Source: CAD feature listing. Evaluate the final solid. Frame: model axes, mm. A direction names the side the tool comes from. Give positions to 0.01 mm unless a question says otherwise; leave off trailing zeros. Write each loop counter-clockwise with the first axis right and the second up, starting at its lowest first coordinate (ties: lowest second). Pieces come first, ordered by that corner, then holes.
```python
from build123d import *

# Parameters (mm, degrees)
RESSALTO_EXTRUS_O1_DEPTH             = 3
ESBO_O2_R                            = 4
CORTE_EXTRUS_O1_DEPTH                = 10
ESCAREADO_PARA_SFHCS_M31_AT_2_COUNT  = 2
ESCAREADO_PARA_SFHCS_M31_AT_2_PITCH  = 110.302460898
ESCAREADO_PARA_SFHCS_M31_AT_3_COUNT  = 2
ESCAREADO_PARA_SFHCS_M31_AT_3_PITCH  = 130.842986965
ESCAREADO_PARA_SFHCS_M31_AT_4_COUNT  = 2
ESCAREADO_PARA_SFHCS_M31_AT_4_PITCH  = 67
ESCAREADO_PARA_SFHCS_M31_AT_5_COUNT  = 2
ESCAREADO_PARA_SFHCS_M31_AT_5_PITCH  = 132.532334398
ESCAREADO_PARA_SFHCS_M31_AT_6_COUNT  = 2
ESCAREADO_PARA_SFHCS_M31_AT_6_PITCH  = 175.070818678
ESCAREADO_PARA_SFHCS_M31_AT_7_COUNT  = 2
ESCAREADO_PARA_SFHCS_M31_AT_7_PITCH  = 213.572320447
ESCAREADO_PARA_SFHCS_M31_AT_8_COUNT  = 2
ESCAREADO_PARA_SFHCS_M31_AT_8_PITCH  = 243.433045731
ESCAREADO_PARA_SFHCS_M31_AT_9_COUNT  = 2
ESCAREADO_PARA_SFHCS_M31_AT_9_PITCH  = 142.710342559
ESCAREADO_PARA_SFHCS_M41_AT_2_COUNT  = 2
ESCAREADO_PARA_SFHCS_M41_AT_2_PITCH  = 40
ESCAREADO_PARA_SFHCS_M41_AT_3_COUNT  = 2
ESCAREADO_PARA_SFHCS_M41_AT_3_PITCH  = 46.75082887
ESCAREADO_PARA_SFHCS_M41_AT_4_COUNT  = 2
ESCAREADO_PARA_SFHCS_M41_AT_4_PITCH  = 24.2
ESCAREADO_PARA_SFHCS_M41_AT_5_COUNT  = 2
ESCAREADO_PARA_SFHCS_M41_AT_5_PITCH  = 58.077850276
ESCAREADO_PARA_SFHCS_M41_AT_6_COUNT  = 2
ESCAREADO_PARA_SFHCS_M41_AT_6_PITCH  = 43.020334562
ESCAREADO_PARA_SFHCS_M41_AT_7_COUNT  = 2
ESCAREADO_PARA_SFHCS_M41_AT_7_PITCH  = 136.807623633
ESCAREADO_PARA_SFHCS_M41_AT_8_COUNT  = 2
ESCAREADO_PARA_SFHCS_M41_AT_8_PITCH  = 139.831145131
ESCAREADO_PARA_SFHCS_M41_AT_9_COUNT  = 2
ESCAREADO_PARA_SFHCS_M41_AT_9_PITCH  = 173.161507104
ESCAREADO_PARA_SFHCS_M41_AT_10_COUNT = 2
ESCAREADO_PARA_SFHCS_M41_AT_10_PITCH = 170.775968029
ESCAREADO_PARA_SFHCS_M41_AT_11_COUNT = 2
ESCAREADO_PARA_SFHCS_M41_AT_11_PITCH = 332.816318971
ESCAREADO_PARA_SFHCS_M41_AT_12_COUNT = 2
ESCAREADO_PARA_SFHCS_M41_AT_12_PITCH = 333.669600313
ESCAREADO_PARA_SFHCS_M41_AT_13_COUNT = 2
ESCAREADO_PARA_SFHCS_M41_AT_13_PITCH = 373.827719057
ESCAREADO_PARA_SFHCS_M41_AT_14_COUNT = 2
ESCAREADO_PARA_SFHCS_M41_AT_14_PITCH = 373.066299115
ESBO_O9_W                            = 8
ESBO_O9_H                            = 4
CORTE_EXTRUS_O2_DEPTH                = 230.077241914


with BuildPart() as part:
    # Esboço1 → Ressalto-extrusão1 (new body)
    with BuildSketch(Plane(origin=(0, 0, 0), x_dir=(1, 0, 0), z_dir=(0, 1, 0))):
        with BuildLine():
            Line((-2.5, 209.375), (2.5, 209.375))
            ThreePointArc((2.5, 209.375), (3.560660172, 209.814339828), (4, 210.875))
            Line((4, 210.875), (4, 213.875))
            ThreePointArc((4, 213.875), (4.439339828, 214.935660172), (5.5, 215.375))
            Line((5.5, 215.375), (21, 215.375))
            ThreePointArc((21, 215.375), (23.121320344, 214.496320344), (24, 212.375))
            Line((24, 212.375), (24, 187.375))
            Line((24, 187.375), (35.808734273, 177.675))
            ThreePointArc((35.808734273, 177.675), (37.1583493, 172.791760303), (33.015886264, 169.875))
            Line((33.015886264, 169.875), (31, 169.875))
            ThreePointArc((31, 169.875), (28.878679656, 168.996320344), (28, 166.875))
            Line((28, 166.875), (28, 155.375))
            Line((28, 155.375), (66.5, 111.375))
            Line((66.5, 111.375), (59.5, -111.375))
            Line((59.5, -111.375), (48, -117.875))
            Line((48, -117.875), (29, -154.770121629))
            Line((29, -154.770121629), (29, -166.370121629))
            ThreePointArc((29, -166.370121629), (29.878679656, -168.491441972), (32, -169.370121629))
            Line((32, -169.370121629), (32.371701685, -169.370121629))
            ThreePointArc((32.371701685, -169.370121629), (36.448422746, -171.9647751), (35.823953384, -176.756634787))
            Line((35.823953384, -176.756634787), (22.5, -192.691999769))
            Line((22.5, -192.691999769), (22.5, -216.191999769))
            ThreePointArc((22.5, -216.191999769), (21.621320344, -218.313320113), (19.5, -219.191999769))
            Line((19.5, -219.191999769), (-19.5, -219.191999769))
            ThreePointArc((-19.5, -219.191999769), (-21.621320344, -218.313320113), (-22.5, -216.191999769))
            Line((-22.5, -216.191999769), (-22.5, -192.691999769))
            Line((-22.5, -192.691999769), (-35.823953384, -176.756634787))
            ThreePointArc((-35.823953384, -176.756634787), (-36.448422746, -171.9647751), (-32.371701685, -169.370121629))
            Line((-32.371701685, -169.370121629), (-32, -169.370121629))
            ThreePointArc((-32, -169.370121629), (-29.878679656, -168.491441972), (-29, -166.370121629))
            Line((-29, -166.370121629), (-29, -154.770121629))
            Line((-29, -154.770121629), (-48, -117.875))
            Line((-48, -117.875), (-59.5, -111.375))
            Line((-59.5, -111.375), (-66.5, 111.375))
            Line((-66.5, 111.375), (-28, 155.375))
            Line((-28, 155.375), (-28, 166.875))
            ThreePointArc((-28, 166.875), (-28.878679656, 168.996320344), (-31, 169.875))
            Line((-31, 169.875), (-33.015886264, 169.875))
            ThreePointArc((-33.015886264, 169.875), (-37.1583493, 172.791760303), (-35.808734273, 177.675))
            Line((-35.808734273, 177.675), (-24, 187.375))
            Line((-24, 187.375), (-24, 212.375))
            ThreePointArc((-24, 212.375), (-23.121320344, 214.496320344), (-21, 215.375))
            Line((-21, 215.375), (-5.5, 215.375))
            ThreePointArc((-5.5, 215.375), (-4.439339828, 214.935660172), (-4, 213.875))
            Line((-4, 213.875), (-4, 210.875))
            ThreePointArc((-4, 210.875), (-3.560660172, 209.814339828), (-2.5, 209.375))
        make_face()
    extrude(amount=RESSALTO_EXTRUS_O1_DEPTH)

    # Esboço2 → Corte-extrusão1 (cut)
    with BuildSketch(Plane(origin=(0, 3, 0), x_dir=(1, 0, 0), z_dir=(0, 1, 0))):
        with Locations(Location((-45, -79.191999769, 0), (0, 0, 270))):
            Circle(ESBO_O2_R)
        with Locations(Location((45, -79.191999769, 0), (0, 0, 270))):
            Circle(ESBO_O2_R)
        with Locations(Location((45, 110.808000231, 0), (0, 0, 270))):
            Circle(ESBO_O2_R)
        with Locations(Location((-45, 110.808000231, 0), (0, 0, 270))):
            Circle(ESBO_O2_R)
    extrude(amount=-CORTE_EXTRUS_O1_DEPTH, mode=Mode.SUBTRACT)

    # Esboço6 → Escareado para SFHCS M31 (revolve, cut)
    with BuildSketch(Plane(origin=(55.151230449, 0, 106.491941439), x_dir=(0, 0, -1), z_dir=(1, 0, 0))):
        Polygon((0, 0), (0, 3), (1.7, 3), (1.7, 1.66), (3.36, 0), align=None)
    escareado_para_sfhcs_m31 = revolve(axis=Axis((55.151230449, -6.35, 106.491941439), (0, 1, 0)), mode=Mode.SUBTRACT)

    # Escareado para SFHCS M31 at 2: Escareado para SFHCS M31 ×2
    with Locations(*[(-i * ESCAREADO_PARA_SFHCS_M31_AT_2_PITCH, 0, 0) for i in range(1, ESCAREADO_PARA_SFHCS_M31_AT_2_COUNT)]):
        add(escareado_para_sfhcs_m31, mode=Mode.SUBTRACT)

    # Escareado para SFHCS M31 at 3: Escareado para SFHCS M31 ×2
    with Locations(*[Vector(-0.8590977939862314, 0, -0.5118114695549434) * (i * ESCAREADO_PARA_SFHCS_M31_AT_3_PITCH) for i in range(1, ESCAREADO_PARA_SFHCS_M31_AT_3_COUNT)]):
        add(escareado_para_sfhcs_m31, mode=Mode.SUBTRACT)

    # Escareado para SFHCS M31 at 4: Escareado para SFHCS M31 ×2
    with Locations(*[Vector(0.031409859126967435, 0, -0.9995065886474306) * (i * ESCAREADO_PARA_SFHCS_M31_AT_4_PITCH) for i in range(1, ESCAREADO_PARA_SFHCS_M31_AT_4_COUNT)]):
        add(escareado_para_sfhcs_m31, mode=Mode.SUBTRACT)

    # Escareado para SFHCS M31 at 5: Escareado para SFHCS M31 ×2
    with Locations(*[Vector(0.03140985912696758, 0, -0.9995065886474307) * (i * ESCAREADO_PARA_SFHCS_M31_AT_5_PITCH) for i in range(1, ESCAREADO_PARA_SFHCS_M31_AT_5_COUNT)]):
        add(escareado_para_sfhcs_m31, mode=Mode.SUBTRACT)

    # Escareado para SFHCS M31 at 6: Escareado para SFHCS M31 ×2
    with Locations(*[Vector(-0.6538227427961019, 0, -0.7566477522616337) * (i * ESCAREADO_PARA_SFHCS_M31_AT_6_PITCH) for i in range(1, ESCAREADO_PARA_SFHCS_M31_AT_6_COUNT)]):
        add(escareado_para_sfhcs_m31, mode=Mode.SUBTRACT)

    # Escareado para SFHCS M31 at 7: Escareado para SFHCS M31 ×2
    with Locations(*[Vector(0.03140985912696757, 0, -0.9995065886474307) * (i * ESCAREADO_PARA_SFHCS_M31_AT_7_PITCH) for i in range(1, ESCAREADO_PARA_SFHCS_M31_AT_7_COUNT)]):
        add(escareado_para_sfhcs_m31, mode=Mode.SUBTRACT)

    # Escareado para SFHCS M31 at 8: Escareado para SFHCS M31 ×2
    with Locations(*[Vector(-0.4806690769772822, 0, -0.8769020688981225) * (i * ESCAREADO_PARA_SFHCS_M31_AT_8_PITCH) for i in range(1, ESCAREADO_PARA_SFHCS_M31_AT_8_COUNT)]):
        add(escareado_para_sfhcs_m31, mode=Mode.SUBTRACT)

    # Escareado para SFHCS M31 at 9: Escareado para SFHCS M31 ×2
    with Locations(*[Vector(-0.3228941175011494, 0, -0.9464350949130923) * (i * ESCAREADO_PARA_SFHCS_M31_AT_9_PITCH) for i in range(1, ESCAREADO_PARA_SFHCS_M31_AT_9_COUNT)]):
        add(escareado_para_sfhcs_m31, mode=Mode.SUBTRACT)

    # Esboço8 → Escareado para SFHCS M41 (revolve, cut)
    with BuildSketch(Plane(origin=(12.1, 0, 170.191999769), x_dir=(0, 0, -1), z_dir=(1, 0, 0))):
        Polygon((0, 0), (0, 3), (2.25, 3), (2.25, 2.23), (4.48, 0), align=None)
    escareado_para_sfhcs_m41 = revolve(axis=Axis((12.1, -6.35, 170.191999769), (0, 1, 0)), mode=Mode.SUBTRACT)

    # Escareado para SFHCS M41 at 2: Escareado para SFHCS M41 ×2
    with Locations(*[(0, 0, i * ESCAREADO_PARA_SFHCS_M41_AT_2_PITCH) for i in range(1, ESCAREADO_PARA_SFHCS_M41_AT_2_COUNT)]):
        add(escareado_para_sfhcs_m41, mode=Mode.SUBTRACT)

    # Escareado para SFHCS M41 at 3: Escareado para SFHCS M41 ×2
    with Locations(*[Vector(-0.5176378811907321, 0, 0.8555998036210444) * (i * ESCAREADO_PARA_SFHCS_M41_AT_3_PITCH) for i in range(1, ESCAREADO_PARA_SFHCS_M41_AT_3_COUNT)]):
        add(escareado_para_sfhcs_m41, mode=Mode.SUBTRACT)

    # Escareado para SFHCS M41 at 4: Escareado para SFHCS M41 ×2
    with Locations(*[(-i * ESCAREADO_PARA_SFHCS_M41_AT_4_PITCH, 0, 0) for i in range(1, ESCAREADO_PARA_SFHCS_M41_AT_4_COUNT)]):
        add(escareado_para_sfhcs_m41, mode=Mode.SUBTRACT)

    # Escareado para SFHCS M41 at 5: Escareado para SFHCS M41 ×2
    with Locations(*[Vector(-0.7498938236983096, 0, -0.6615582009008192) * (i * ESCAREADO_PARA_SFHCS_M41_AT_5_PITCH) for i in range(1, ESCAREADO_PARA_SFHCS_M41_AT_5_COUNT)]):
        add(escareado_para_sfhcs_m41, mode=Mode.SUBTRACT)

    # Escareado para SFHCS M41 at 6: Escareado para SFHCS M41 ×2
    with Locations(*[Vector(0.44983892878661463, 0, -0.8931097010715487) * (i * ESCAREADO_PARA_SFHCS_M41_AT_6_PITCH) for i in range(1, ESCAREADO_PARA_SFHCS_M41_AT_6_COUNT)]):
        add(escareado_para_sfhcs_m41, mode=Mode.SUBTRACT)

    # Escareado para SFHCS M41 at 7: Escareado para SFHCS M41 ×2
    with Locations(*[Vector(-0.039657765677978324, 0, -0.999213321379089) * (i * ESCAREADO_PARA_SFHCS_M41_AT_7_PITCH) for i in range(1, ESCAREADO_PARA_SFHCS_M41_AT_7_COUNT)]):
        add(escareado_para_sfhcs_m41, mode=Mode.SUBTRACT)

    # Escareado para SFHCS M41 at 8: Escareado para SFHCS M41 ×2
    with Locations(*[Vector(-0.21043584140980087, 0, -0.9776076701060344) * (i * ESCAREADO_PARA_SFHCS_M41_AT_8_PITCH) for i in range(1, ESCAREADO_PARA_SFHCS_M41_AT_8_COUNT)]):
        add(escareado_para_sfhcs_m41, mode=Mode.SUBTRACT)

    # Escareado para SFHCS M41 at 9: Escareado para SFHCS M41 ×2
    with Locations(*[Vector(-0.16801225891576932, 0, -0.9857849059779829) * (i * ESCAREADO_PARA_SFHCS_M41_AT_9_PITCH) for i in range(1, ESCAREADO_PARA_SFHCS_M41_AT_9_COUNT)]):
        add(escareado_para_sfhcs_m41, mode=Mode.SUBTRACT)

    # Escareado para SFHCS M41 at 10: Escareado para SFHCS M41 ×2
    with Locations(*[Vector(-0.0298241961363705, 0, -0.9995551597209728) * (i * ESCAREADO_PARA_SFHCS_M41_AT_10_PITCH) for i in range(1, ESCAREADO_PARA_SFHCS_M41_AT_10_COUNT)]):
        add(escareado_para_sfhcs_m41, mode=Mode.SUBTRACT)

    # Escareado para SFHCS M41 at 11: Escareado para SFHCS M41 ×2
    with Locations(*[Vector(-0.0010516311251878737, 0, -0.9999994470358354) * (i * ESCAREADO_PARA_SFHCS_M41_AT_11_PITCH) for i in range(1, ESCAREADO_PARA_SFHCS_M41_AT_11_COUNT)]):
        add(escareado_para_sfhcs_m41, mode=Mode.SUBTRACT)

    # Escareado para SFHCS M41 at 12: Escareado para SFHCS M41 ×2
    with Locations(*[Vector(-0.0714778930343451, 0, -0.9974421841928337) * (i * ESCAREADO_PARA_SFHCS_M41_AT_12_PITCH) for i in range(1, ESCAREADO_PARA_SFHCS_M41_AT_12_COUNT)]):
        add(escareado_para_sfhcs_m41, mode=Mode.SUBTRACT)

    # Escareado para SFHCS M41 at 13: Escareado para SFHCS M41 ×2
    with Locations(*[Vector(-0.06379944232106374, 0, -0.9979627403663532) * (i * ESCAREADO_PARA_SFHCS_M41_AT_13_PITCH) for i in range(1, ESCAREADO_PARA_SFHCS_M41_AT_13_COUNT)]):
        add(escareado_para_sfhcs_m41, mode=Mode.SUBTRACT)

    # Escareado para SFHCS M41 at 14: Escareado para SFHCS M41 ×2
    with Locations(*[Vector(-0.0009381710458172143, 0, -0.9999995599174476) * (i * ESCAREADO_PARA_SFHCS_M41_AT_14_PITCH) for i in range(1, ESCAREADO_PARA_SFHCS_M41_AT_14_COUNT)]):
        add(escareado_para_sfhcs_m41, mode=Mode.SUBTRACT)

    # Esboço9 → Corte-extrusão2 (cut, through all)
    with BuildSketch(Plane.XZ):
        with BuildLine():
            Line((-13.794262039, 13.491999769), (2.205737961, 13.491999769))
            ThreePointArc((2.205737961, 13.491999769), (7.205737961, 8.491999769), (2.205737961, 3.491999769))
            Line((2.205737961, 3.491999769), (-13.794262039, 3.491999769))
            ThreePointArc((-13.794262039, 3.491999769), (-18.794262039, 8.491999769), (-13.794262039, 13.491999769))
        make_face()
        with Locations((0.15, -151.574135166)):
            Rectangle(ESBO_O9_W, ESBO_O9_H)
    extrude(amount=-CORTE_EXTRUS_O2_DEPTH, mode=Mode.SUBTRACT)


solid = part.part
```
1. Contact query for flat-ended pins moving along their axis: P1, Ø4, axis at x = -59.31, z = -25.98, coming from the -Y side; P2, Ø0.9, axis at y = 2, z = -203.5, coming from the -X side; P3, Ø1.5, axis at y = 1, z = -147.5, coming from the +X side; P4, Ø4, axis at x = 12.1, z = 210.192, coming from the -Y side. Output: stop coordinate, or through.
2. Cut plane A-A, the plane z = -120. Return the cut outline in (x, y).
3. Mould query, pull axis Z, two halves, no side actions, for faces 1 (the conical face through (-14.87, 2.09, -1.61)), 2 (the flat face through (-29.987, 1.479, -182.457)), 3 (the flat face through (-29.1, 1.5, 184.8)). Classes: +Z half, -Z half, draft (parallel to the pull), parting line (faces both ways), or undercut.
4. Cut plane B-B, the plane y = 0.7. State how many separate pieces and enclosed holes the cut face has, then the cut area to 3 significant figures.
5. Access query for faces 4 (the flat face through (-38.367, 1.479, 136.581)), 5 (the conical face through (11.032, 2.091, -164.903)). Directions: +Z, -Z, +X, -X, +Y, -Y. A direction counts if a zero-diameter tool reaches every point of the face in a straight line with its end or side. Return the directions, or none.
6. Line query: L1, parallel to X at y = 0.85, z = -165.5; L2, parallel to Z at x = 35, y = 2.45 (3 decimals); L3, parallel to Z at x = -48.5, y = 1.35. Output: solid intervals per line, ascending.
7. Cut plane C-C, the plane z = 50. Return the cut outline in (x, y), then the cut area to 3 significant figures.
Response values:
1. P1: stops at y = 1.35
1. P2: stops at x = -24
1. P3: stops at x = 35.55
1. P4: passes through
2. outline: (-58.95, 0) - (58.95, 0) - (58.95, 3) - (-58.95, 3) - close
3. face 1: undercut
3. face 2: -Z half
3. face 3: +Z half
4. separate pieces: 1
4. enclosed holes: 29
4. area: 41,200 mm2
5. face 4: -X, +Y, -Y
5. face 5: -Y
6. L1: x = -28 to -13.97, -9.53 to 9.53, 13.97 to 28
6. L2: z = -178.339 to -170.348, -147.375 to 143.119, 170.217 to 177.742
6. L3: z = -131.95 to -112.74, -108.87 to 77.26, 81.13 to 117.59
7. outline: (-61.43, 0) - (61.43, 0) - (61.43, 3) - (-61.43, 3) - close
7. area: 369 mm2
